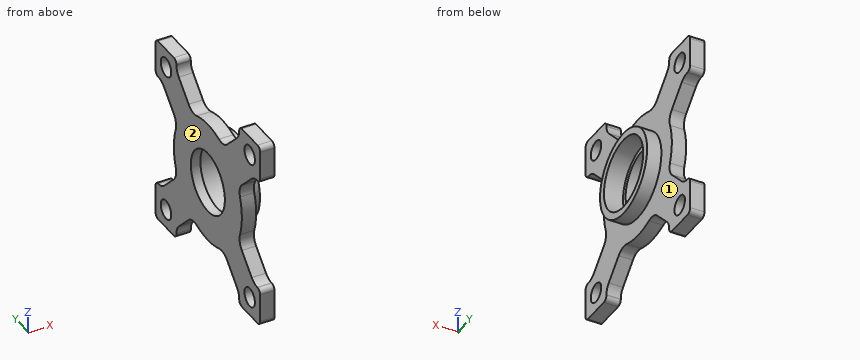
from build123d import *

# Parameters (mm, degrees)
SKETCH_1_R          = 2
EXTRUDE_1_DEPTH     = 3
SKETCH_2_R          = 9
EXTRUDE_2_DEPTH     = 3
SKETCH_3_R          = 7.5
CUT_EXTRUDE_1_DEPTH = 4
SKETCH_4_R          = 6.5
CUT_EXTRUDE_2_DEPTH = 57.709787515


with BuildPart() as part:
    # 草图1 → 凸台-拉伸1 (new body)
    with BuildSketch(Plane(origin=(0, 0, 0), x_dir=(0, 0, -1), z_dir=(1, 0, 0))):
        with BuildLine():
            Line((1, 0), (7, 0))
            ThreePointArc((7, 0), (7.707106781, -0.292893219), (8, -1))
            Line((8, -1), (8, -1.100505063))
            ThreePointArc((8, -1.100505063), (8.228361402, -2.24855536), (8.878679656, -3.221825407))
            Line((8.878679656, -3.221825407), (12.65493215, -6.998077901))
            ThreePointArc((12.65493215, -6.998077901), (14.102815672, -7.800194378), (15.755705151, -7.712365515))
            ThreePointArc((15.755705151, -7.712365515), (20, -7), (24.244294849, -7.712365515))
            ThreePointArc((24.244294849, -7.712365515), (25.897184328, -7.800194378), (27.34506785, -6.998077901))
            Line((27.34506785, -6.998077901), (31.121320344, -3.221825407))
            ThreePointArc((31.121320344, -3.221825407), (31.771638598, -2.24855536), (32, -1.100505063))
            Line((32, -1.100505063), (32, -1))
            ThreePointArc((32, -1), (32.292893219, -0.292893219), (33, 0))
            Line((33, 0), (39, 0))
            ThreePointArc((39, 0), (39.707106781, -0.292893219), (40, -1))
            Line((40, -1), (40, -7))
            ThreePointArc((40, -7), (39.707106781, -7.707106781), (39, -8))
            Line((39, -8), (38.899494937, -8))
            ThreePointArc((38.899494937, -8), (37.75144464, -8.228361402), (36.778174593, -8.878679656))
            Line((36.778174593, -8.878679656), (33.001922099, -12.65493215))
            ThreePointArc((33.001922099, -12.65493215), (32.199805622, -14.102815672), (32.287634485, -15.755705151))
            ThreePointArc((32.287634485, -15.755705151), (33, -20), (32.287634485, -24.244294849))
            ThreePointArc((32.287634485, -24.244294849), (32.199805622, -25.897184328), (33.001922099, -27.34506785))
            Line((33.001922099, -27.34506785), (36.778174593, -31.121320344))
            ThreePointArc((36.778174593, -31.121320344), (37.75144464, -31.771638598), (38.899494937, -32))
            Line((38.899494937, -32), (39, -32))
            ThreePointArc((39, -32), (39.707106781, -32.292893219), (40, -33))
            Line((40, -33), (40, -39))
            ThreePointArc((40, -39), (39.707106781, -39.707106781), (39, -40))
            Line((39, -40), (33, -40))
            ThreePointArc((33, -40), (32.292893219, -39.707106781), (32, -39))
            Line((32, -39), (32, -38.899494937))
            ThreePointArc((32, -38.899494937), (31.771638598, -37.75144464), (31.121320344, -36.778174593))
            Line((31.121320344, -36.778174593), (27.34506785, -33.001922099))
            ThreePointArc((27.34506785, -33.001922099), (25.897184328, -32.199805622), (24.244294849, -32.287634485))
            ThreePointArc((24.244294849, -32.287634485), (20, -33), (15.755705151, -32.287634485))
            ThreePointArc((15.755705151, -32.287634485), (14.102815672, -32.199805622), (12.65493215, -33.001922099))
            Line((12.65493215, -33.001922099), (8.878679656, -36.778174593))
            ThreePointArc((8.878679656, -36.778174593), (8.228361402, -37.75144464), (8, -38.899494937))
            Line((8, -38.899494937), (8, -39))
            ThreePointArc((8, -39), (7.707106781, -39.707106781), (7, -40))
            Line((7, -40), (1, -40))
            ThreePointArc((1, -40), (0.292893219, -39.707106781), (0, -39))
            Line((0, -39), (0, -33))
            ThreePointArc((0, -33), (0.292893219, -32.292893219), (1, -32))
            Line((1, -32), (1.100505063, -32))
            ThreePointArc((1.100505063, -32), (2.24855536, -31.771638598), (3.221825407, -31.121320344))
            Line((3.221825407, -31.121320344), (6.998077901, -27.34506785))
            ThreePointArc((6.998077901, -27.34506785), (7.800194378, -25.897184328), (7.712365515, -24.244294849))
            ThreePointArc((7.712365515, -24.244294849), (7, -20), (7.712365515, -15.755705151))
            ThreePointArc((7.712365515, -15.755705151), (7.800194378, -14.102815672), (6.998077901, -12.65493215))
            Line((6.998077901, -12.65493215), (3.221825407, -8.878679656))
            ThreePointArc((3.221825407, -8.878679656), (2.24855536, -8.228361402), (1.100505063, -8))
            Line((1.100505063, -8), (1, -8))
            ThreePointArc((1, -8), (0.292893219, -7.707106781), (0, -7))
            Line((0, -7), (0, -1))
            ThreePointArc((0, -1), (0.292893219, -0.292893219), (1, 0))
        make_face()
        with Locations((4, -4)):
            Circle(SKETCH_1_R, mode=Mode.SUBTRACT)
        with Locations((36, -4)):
            Circle(SKETCH_1_R, mode=Mode.SUBTRACT)
        with Locations((4, -36)):
            Circle(SKETCH_1_R, mode=Mode.SUBTRACT)
        with Locations((36, -36)):
            Circle(SKETCH_1_R, mode=Mode.SUBTRACT)
    extrude(amount=EXTRUDE_1_DEPTH)

    # 草图2 → 凸台-拉伸2 (add)
    with BuildSketch(Plane(origin=(3, 0, 0), x_dir=(0, 0, -1), z_dir=(1, 0, 0))):
        with Locations((20, -20)):
            Circle(SKETCH_2_R)
    extrude(amount=EXTRUDE_2_DEPTH)

    # 草图3 → 切除-拉伸1 (cut)
    with BuildSketch(Plane(origin=(6, 0, 0), x_dir=(0, 0, -1), z_dir=(1, 0, 0))):
        with Locations((20, -20)):
            Circle(SKETCH_3_R)
    extrude(amount=-CUT_EXTRUDE_1_DEPTH, mode=Mode.SUBTRACT)

    # 草图4 → 切除-拉伸2 (cut, through all)
    with BuildSketch(Plane(origin=(2, 0, 0), x_dir=(0, 0, -1), z_dir=(1, 0, 0))):
        with Locations((20, -20)):
            Circle(SKETCH_4_R)
    extrude(amount=-CUT_EXTRUDE_2_DEPTH, mode=Mode.SUBTRACT)


solid = part.part
Could you check a few things on this model? Use its own coordinates, in mm. Face numbers are marked on the shaded views. A direction names the side the tool comes from. Give positions to 0.01 mm unless a question says otherwise; leave off trailing zeros. Write each loop counter-clockwise with the first axis right and the second up, starting at its lowest first coordinate (ties: lowest second). Pieces come first, ordered by that corner, then holes. Notation, with made-up numbers: (86.25, -38.5) - (108.25, -38.5) arc R22 ccw to (108.25, 0.5) - close; hole circle Ø2 at (-35, -10). An arc over 180 degrees is marked (long way). Use CSV: the item, a comma, the result in double quotes. Start each with the question number.
Item 1: I want a section at C-C, the plane x = 5.5. Please give me the cut outline in (y, z), then the cut area to 3 significant figures.
Item 2: I'm going to push flat-ended pins straight in: pin 1 (12 mm diameter, centred on y = -18, z = -21.5, fed in from +X); pin 2 (1.5 mm diameter, centred on x = 2, z = -17, fed in from -Y); pin 3 (6 mm diameter, centred on y = -21.5, z = -7, fed in from +X); pin 4 (3 mm diameter, centred on x = 1.5, z = -29, fed in from +Y). Where does each tip first touch, or does it pass through?
Item 3: I want a section at A-A, the plane y = -20. Please give me the cut outline in (x, z), then the cut area to 3 significant figures.
Item 4: For the marked faces 1 and 2, which set-ups out of +Z, -Z, +X, -X, +Y, -Y let a thin tool reach every point of the face, with its end or its side?
Item 5: I want a section at D-D, the plane z = -36. Please give me the cut outline in (x, y), then the cut area to 3 significant figures.
Item 6: If I drill on line 1 along Y through (x, z) = (1.35, -36); line 2 along Y through (x, z) = (1.3, -5.5); line 3 along Y through (x, z) = (2.95, -20), over which ranges is the centre line in solid material (lowest first)?
Findings:
1,outline,"circle Ø18 at (-20, -20); hole circle Ø15 at (-20, -20)"
1,area,"77.8 mm2"
2,pin 1,"stops at x = 6"
2,pin 2,"stops at y = -32.8"
2,pin 3,"stops at x = 3"
2,pin 4,"stops at y = -3.84"
3,outline,"(0, -33) - (3, -33) - (3, -29) - (6, -29) - (6, -27.5) - (2, -27.5) - (2, -26.5) - (0, -26.5) - close; (0, -13.5) - (2, -13.5) - (2, -12.5) - (6, -12.5) - (6, -11) - (3, -11) - (3, -7) - (0, -7) - close"
3,area,"46.0 mm2"
4,face 1,"+X"
4,face 2,"+Z, -Z, -X, +Y, -Y"
5,outline,"(0, -40) - (3, -40) - (3, -38) - (0, -38) - close; (0, -34) - (3, -34) - (3, -30.34) - (0, -30.34) - close; (0, -9.66) - (3, -9.66) - (3, -6) - (0, -6) - close; (0, -2) - (3, -2) - (3, 0) - (0, 0) - close"
5,area,"33.9 mm2"
6,line 1,"y = -40 to -38, -34 to -30.34, -9.66 to -6, -2 to 0"
6,line 2,"y = -40 to -37.32, -34.68 to -28.84, -11.16 to -5.32, -2.68 to 0"
6,line 3,"y = -33 to -27.5, -12.5 to -7"
